Answer from the drawing. Dimensions are ordinates in mm from the lowest x, y and z of the part. A direction names the side the tool comes from. Give positions to 0.01 mm unless a question says otherwise; leave off trailing zeros. Write each loop counter-clockwise with the first axis right and the second up, starting at its lowest first coordinate (ties: lowest second). Pieces come first, ordered by that corner, then holes. Notation, with made-up numbers: M -17.5,61.25 L -4.5,61.25 A32 cw -4.5,93.25 Z; hole C 32,37 d10. An arc over 180 degrees is marked long. Answer as a JSON object with one key per item and string values.
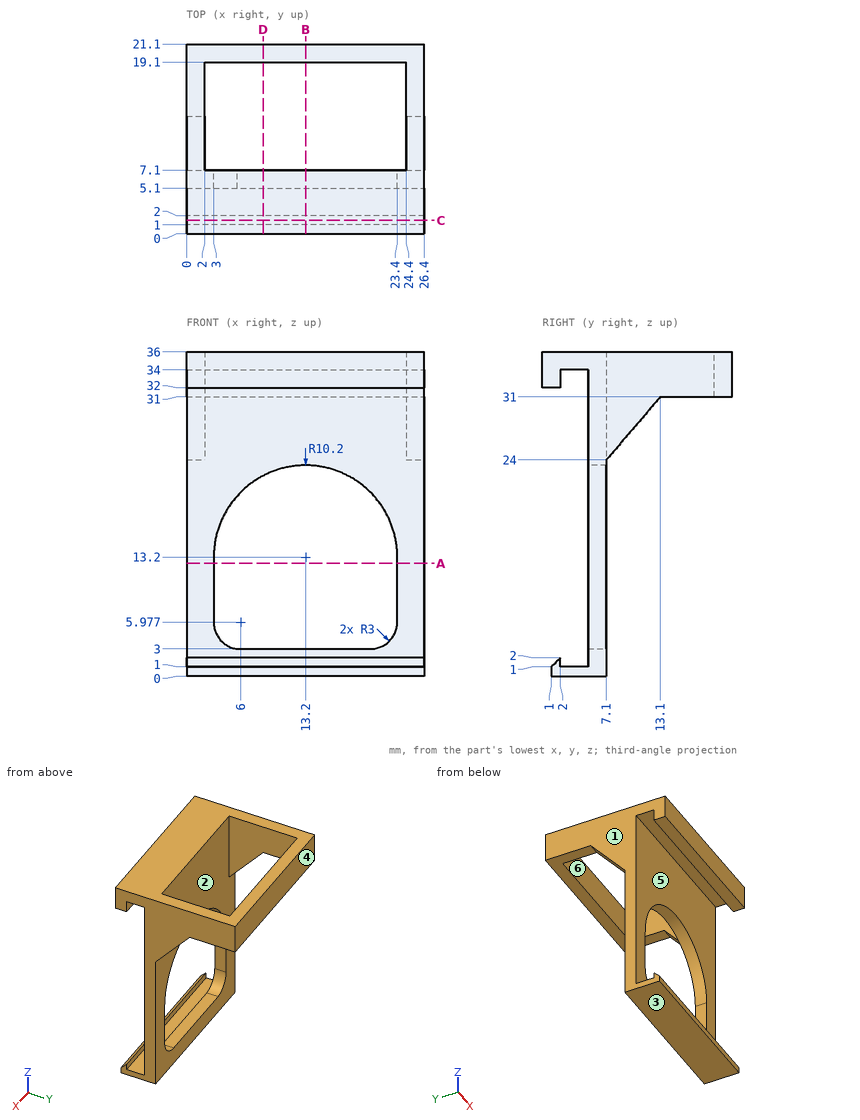
1. Consider line 1 along Y through (x, z) = (14, 33); line 2 along Z through (x, y) = (4.5, 4); line 3 along X through (y, z) = (17.5, 34.5). Determine where each line is inside the solid, lowest interval first.
Verdict:
{"line 1": "y = 0 to 2, 5.1 to 7.1, 19.1 to 21.1", "line 2": "z = 0 to 1, 34 to 36", "line 3": "x = 0 to 2, 24.4 to 26.4"}
2. A cutting plane is placed at A-A, the plane z = 12.5. Give the vertices of the cut face in (x, y), plus the area to 3 significant figures.
Verdict:
{"outline": "M 0,5.1 L 3,5.1 L 3,7.1 L 0,7.1 Z; M 23.4,5.1 L 26.4,5.1 L 26.4,7.1 L 23.4,7.1 Z", "area": "12.0 mm2"}
3. Flat-ended cylindrical pins translate along their axes: pin 1 (10 mm diameter, centred on x = 4.5, y = 5, fed in from -Z); pin 2 (6.5 mm diameter, centred on x = 17.5, y = 17.5, fed in from -Z); pin 3 (6 mm diameter, centred on x = 7, z = 12.5, fed in from -Y); pin 4 (0.8 mm diameter, centred on x = 19.5, z = 0.5, fed in from -Y). Find the tip coordinate at first contact, or state that the pin passes through.
Verdict:
{"pin 1": "stops at z = 0", "pin 2": "stops at z = 31", "pin 3": "passes through", "pin 4": "stops at y = 1"}
4. For the marked faces 4, 5 and 6, determine the directions among +Z, -Z, +X, -X, +Y, -Y from which every point of the face is accessible in a straight line to the end or side of a thin tool.
Verdict:
{"face 4": "+Z, -Z, +X, -X, +Y", "face 5": "+X, -X", "face 6": "+Z, -Z"}
5. The mould has two halves that part along X. Classify the marked faces 1, 2 and 3: released by +X, released by -X, zero draft, split by the parting line, or undercut.
Verdict:
{"face 1": "released by -X", "face 2": "undercut", "face 3": "zero draft"}
6. A cutting plane is placed at D-D, the plane x = 8.5. Give the vertices of the cut face in (y, z).
Verdict:
{"outline": "M 0,32 L 2,32 L 2,34 L 5.1,34 L 5.1,22.25 L 7.1,22.25 L 7.1,36 L 0,36 Z; M 1,0 L 7.1,0 L 7.1,3 L 5.1,3 L 5.1,1 L 2,1 L 2,2 L 1,1 Z; M 19.1,31 L 21.1,31 L 21.1,36 L 19.1,36 Z"}
7. A cutting plane is placed at C-C, the plane y = 1.5. Give the vertices of the cut face in (x, z).
Verdict:
{"outline": "M 0,0 L 26.4,0 L 26.4,1.5 L 0,1.5 Z; M 0,32 L 26.4,32 L 26.4,36 L 0,36 Z"}
8. A cutting plane is placed at B-B, the plane x = 13.2. Give the vertices of the cut face in (y, z), plus the area to 3 significant figures.
Verdict:
{"outline": "M 0,32 L 2,32 L 2,34 L 5.1,34 L 5.1,23.4 L 7.1,23.4 L 7.1,36 L 0,36 Z; M 1,0 L 7.1,0 L 7.1,3 L 5.1,3 L 5.1,1 L 2,1 L 2,2 L 1,1 Z; M 19.1,31 L 21.1,31 L 21.1,36 L 19.1,36 Z", "area": "60.0 mm2"}
